```python
from build123d import *

# Parameters (mm, degrees)
SKETCH_1_W      = 26.2
SKETCH_1_H      = 15.4
SKETCH_1_R      = 1.5
SKETCH_1_W_2    = 25
SKETCH_1_H_2    = 2.55
EXTRUDE_1_DEPTH = 1.6
SKETCH_1_3_W    = 25
SKETCH_1_3_H    = 2.55
EXTRUDE_2_DEPTH = 2.65
SKETCH_2_W      = 0.628205128
SKETCH_2_H      = 3.5
EXTRUDE_3_DEPTH = 1.7


with BuildPart() as part:
    # Sketch 1 → Extrude 1 (new body)
    # profile 1 of 2: a face of its own
    with BuildSketch(Plane(origin=(0, 0, 0), x_dir=(1, 0, 0), z_dir=(0, 1, 0))):
        Rectangle(SKETCH_1_W, SKETCH_1_H)
        with Locations(Location((-10.15, -5.1, 0), (0, 0, 270))):
            Circle(SKETCH_1_R, mode=Mode.SUBTRACT)
        with Locations(Location((10.15, -5.1, 0), (0, 0, 270))):
            Circle(SKETCH_1_R, mode=Mode.SUBTRACT)
        with Locations((0, 6.025)):
            Rectangle(SKETCH_1_W_2, SKETCH_1_H_2, mode=Mode.SUBTRACT)
    # profile 2 of 2: a face of its own
    with BuildSketch(Plane(origin=(0, 0, 0), x_dir=(1, 0, 0), z_dir=(0, 1, 0))):
        with Locations((0, 6.025)):
            Rectangle(SKETCH_1_W_2, SKETCH_1_H_2)
    extrude(amount=EXTRUDE_1_DEPTH)

    # Sketch 1_3 → Extrude 2 (add)
    with BuildSketch(Plane(origin=(0, 0, 0), x_dir=(1, 0, 0), z_dir=(0, 1, 0))):
        with Locations((0, 6.025)):
            Rectangle(SKETCH_1_3_W, SKETCH_1_3_H)
    extrude(amount=-EXTRUDE_2_DEPTH)

    # Sketch 2 → Extrude 3 (add)
    with BuildSketch(Plane(origin=(0, 1.6, 0), x_dir=(1, 0, 0), z_dir=(0, 1, 0))):
        Polygon((0.5, -1.5), (-0.5, -1.5), (-0.5, -5.5), (-1.2, -5.5), (0, -6.930104311), (1.2, -5.5), (0.5, -5.5), align=None)
        Polygon((5.5, -1.2), (6.930104311, 0), (5.5, 1.2), (5.5, 0.5), (1.5, 0.5), (1.5, -0.5), (5.5, -0.5), align=None)
        with Locations((-3.28532471, 3.544331345)):
            Rectangle(SKETCH_2_W, SKETCH_2_H)
        Polygon((-1.886586729, 5.294331345), (-1.23454346, 5.294331345), (-0.435965736, 2.853025255), (0.368220963, 5.294331345), (1.013954136, 5.294331345), (1.605700931, 1.794331345), (0.969783463, 1.794331345), (0.596085547, 4.004968364), (-0.131678877, 1.794331345), (-0.744459325, 1.794331345), (-1.468017018, 4.004968364), (-1.841013812, 1.794331345), (-2.477632402, 1.794331345), align=None)
        with BuildLine():
            Line((2.189034264, 5.294331345), (2.817239393, 5.294331345))
            Line((2.817239393, 5.294331345), (2.817239393, 3.017087755))
            add(Edge.make_bspline(
                [(2.817239393, 3.017087755), (2.817273551, 2.993478281), (2.817339529, 2.947876826), (2.82064238, 2.882453669), (2.823664717, 2.822316089), (2.82911787, 2.767529925), (2.837174047, 2.71807174), (2.844975055, 2.673623833), (2.855532948, 2.634981994), (2.871399773, 2.590997464), (2.895845342, 2.541578443), (2.935788046, 2.490072805), (2.981878508, 2.443066435), (3.037120582, 2.403940113), (3.099207788, 2.372290446), (3.167798984, 2.348841544), (3.242797481, 2.335807069), (3.294654828, 2.333817117), (3.321345963, 2.332792883)],
                knots=[0, 0, 0, 0, 1.155499968, 2.231836252, 3.205919964, 4.102923608, 4.924856345, 5.658536265, 6.31071849, 6.882491295, 7.94666036, 8.992281882, 10.060072772, 11.158554251, 12.289267114, 13.461410017, 14.693379945, 16, 16, 16, 16], degree=3))
            add(Edge.make_bspline(
                [(3.321345963, 2.332792883), (3.349702001, 2.333620333), (3.404991473, 2.33523372), (3.484516578, 2.351070858), (3.558197038, 2.376289005), (3.624472787, 2.412281729), (3.68327787, 2.455425316), (3.733055141, 2.504622525), (3.772339181, 2.55997148), (3.797943056, 2.611035105), (3.812318371, 2.658034726), (3.823093386, 2.700027104), (3.830992664, 2.749573953), (3.838159148, 2.805901493), (3.842465653, 2.869593167), (3.847135356, 2.940136761), (3.848846846, 3.018014951), (3.849138556, 3.072242996), (3.849290675, 3.100521249)],
                knots=[0, 0, 0, 0, 1.261321664, 2.459363699, 3.594844139, 4.716940403, 5.803436589, 6.833651888, 7.818396249, 8.814403945, 9.360733334, 10.004355033, 10.743453831, 11.592799886, 12.532235708, 13.585170094, 14.740740724, 16, 16, 16, 16], degree=3))
            Line((3.849290675, 3.100521249), (3.849290675, 5.294331345))
            Line((3.849290675, 5.294331345), (4.477495803, 5.294331345))
            Line((4.477495803, 5.294331345), (4.477495803, 3.20639064))
            add(Edge.make_bspline(
                [(4.477495803, 3.20639064), (4.477408565, 3.164089061), (4.477240816, 3.08274725), (4.474664688, 2.965853344), (4.469180577, 2.859089511), (4.464574557, 2.762424556), (4.455660331, 2.675988702), (4.446373798, 2.599412843), (4.434537313, 2.532968347), (4.416925335, 2.457329363), (4.386532275, 2.370233842), (4.337534678, 2.269947127), (4.275335399, 2.171760357), (4.201818961, 2.076753656), (4.118812177, 1.988495493), (4.028155486, 1.91101625), (3.931289197, 1.845477164), (3.827201127, 1.793480747), (3.71597986, 1.752927462), (3.596524945, 1.725677696), (3.46891784, 1.707267413), (3.380777201, 1.705498879), (3.335368399, 1.704587755)],
                knots=[0, 0, 0, 0, 1.170808336, 2.251350247, 3.235597562, 4.129743112, 4.929140599, 5.639994148, 6.264258765, 6.79612947, 7.788252245, 8.809469599, 9.879094798, 10.999557536, 12.129761673, 13.226370002, 14.293821979, 15.358369427, 16.438775801, 17.562147481, 18.744053101, 20, 20, 20, 20], degree=3))
            add(Edge.make_bspline(
                [(3.335368399, 1.704587755), (3.305197888, 1.705095937), (3.245672088, 1.706098571), (3.158128956, 1.714939179), (3.073501323, 1.727966912), (2.991948202, 1.746973032), (2.913186538, 1.771525389), (2.837237257, 1.801747631), (2.764382604, 1.837471182), (2.695030264, 1.878367463), (2.62926558, 1.92258975), (2.569160054, 1.971612016), (2.512645313, 2.021808881), (2.461354044, 2.075292841), (2.414901005, 2.131502406), (2.373381866, 2.190564964), (2.33685831, 2.252475271), (2.304411607, 2.318349254), (2.276640395, 2.391535053), (2.253228221, 2.474635914), (2.232774795, 2.568954362), (2.217575015, 2.67470289), (2.203794806, 2.791532964), (2.195072693, 2.919748944), (2.190509763, 3.059354507), (2.189538525, 3.156140151), (2.189034264, 3.20639064)],
                knots=[0, 0, 0, 0, 1.001158378, 1.975264943, 2.917723546, 3.841610987, 4.75185031, 5.653588123, 6.552117133, 7.442167995, 8.324307438, 9.179605724, 10.014504199, 10.831958861, 11.636465792, 12.43274043, 13.225645099, 14.020104002, 14.867201867, 15.819789774, 16.883317127, 18.068162734, 19.364263498, 20.787406516, 22.332041935, 24, 24, 24, 24], degree=3))
            Line((2.189034264, 3.20639064), (2.189034264, 5.294331345))
        make_face()
        Polygon((1.779131112, -4.434974289), (2.226887522, -4.434974289), (2.66913178, -5.114665128), (3.112224061, -4.434974289), (3.560404483, -4.434974289), (2.893009985, -5.458538659), (3.604501705, -6.551640956), (3.156745295, -6.551640956), (2.66913178, -5.801988178), (2.18024623, -6.551640956), (1.732065808, -6.551640956), (2.445253575, -5.458114647), align=None)
        Polygon((6.501577719, -0.872404796), (6.924317436, -0.872404796), (7.302111907, -1.614849374), (7.679906378, -0.872404796), (8.102646095, -0.872404796), (7.492069172, -2.072358055), (7.492069172, -2.989071463), (7.112154642, -2.989071463), (7.112154642, -2.072358055), align=None)
    extrude(amount=EXTRUDE_3_DEPTH)


solid = part.part
```
Geometry check sheet. Reference: the model listing, model coordinates, mm. A direction names the side the tool comes from. Give positions to 0.01 mm unless a question says otherwise; leave off trailing zeros. Order: outer loops, then holes, each group sorted by start corner. A loop starts at its lowest first (then second) coordinate and runs counter-clockwise, first axis right, second up. Notation, with made-up numbers: (-26.5, 15) - (7.5, 15) arc R20 ccw to (7.5, 40) - close; hole circle Ø3 at (8, 60). An arc over 180 degrees is marked (long way). Answer in a Markdown table with one row per item. Add a question column.
Q1. Cross-section at C-C, the plane z = -0.75. Enter the section's corners in (x, y).
Q2. Material ranges on probe 1 along X at (y, z) = (1.25, 5.1); probe 2 along Y at (x, z) = (1, -2.5); probe 3 along Z at (x, y) = (11, -0.3), recorded low to high. Write a range as from..to.
Q3. Mould release check, pull along Z, two halves, no side actions. Record for faces 5 (the flat face through (7.3, 3.3, 1.9)), 6 (the flat face through (0.24, 2.44, -2.92)), 7 (the flat face through (-0.608, 2.438, 6.205)): pulls with the +Z half, pulls with the -Z half, needs draft (parallel to the pull), parting line crosses it, or undercut.
Q4. Tool access check on faces 1 (the flat face through (0, 2, 1.5)), 2 (the flat face through (7.112, 2.4, 2.5)), 3 (the flat face through (1.5, 2, 0)), 4 (the flat face through (-3.599, 2, -4)). Record the directions out of +Z, -Z, +X, -X, +Y, -Y that give a thin tool (end or side, any length) a straight path to the whole face; none if there is none.
Q5. Cross-section at B-B, the plane x = -8. Enter the section's corners in (y, z).
Q6. Gauge pin test, flat ends, axial feed: pin 1 (0.5 mm diameter, centred on x = 7, y = 2.5, fed in from -Z); pin 2 (2 mm diameter, centred on x = 5.5, z = 3, fed in from +Y); pin 3 (5 mm diameter, centred on x = 3.5, z = 1.5, fed in from -Y); pin 4 (2.5 mm diameter, centred on x = -10.15, z = 5.1, fed in from -Y). Record the tip position at first contact, or that the pin passes through.
Q7. Cross-section at D-D, the plane y = -1.95. Enter the section's corners in (x, z), then the cut area to 4 significant figures.
Q8. Cross-section at A-A, the plane x = 10.15. Enter the section's corners in (y, z), then the cut area to 3 significant figures.
Check values:
| question | item | result |
|---|---|---|
| 1 | outline | (-13.1, 0) - (13.1, 0) - (13.1, 1.6) - (6.04, 1.6) - (6.04, 3.3) - (5.5, 3.3) - (5.5, 1.6) - (-13.1, 1.6) - close |
| 2 | probe 1 | x = -13.1..-11.65, -8.65..8.65, 11.65..13.1 |
| 2 | probe 2 | y = 0..3.3 |
| 2 | probe 3 | z = -7.3..-4.75 |
| 3 | face 5 | needs draft |
| 3 | face 6 | undercut |
| 3 | face 7 | pulls with the +Z half |
| 4 | face 1 | -X, +Y |
| 4 | face 2 | +Z, +Y |
| 4 | face 3 | +Z, -X, +Y |
| 4 | face 4 | +Z, -Z, -X, +Y |
| 5 | outline | (-2.65, -7.3) - (0, -7.3) - (0, -7.7) - (1.6, -7.7) - (1.6, 7.7) - (0, 7.7) - (0, -4.75) - (-2.65, -4.75) - close |
| 6 | pin 1 | stops at z = -0.15 |
| 6 | pin 2 | stops at y = 1.6 |
| 6 | pin 3 | stops at y = 0 |
| 6 | pin 4 | passes through |
| 7 | outline | (-12.5, -7.3) - (12.5, -7.3) - (12.5, -4.75) - (-12.5, -4.75) - close |
| 7 | area | 63.75 mm^2 |
| 8 | outline | (-2.65, -7.3) - (0, -7.3) - (0, -7.7) - (1.6, -7.7) - (1.6, 3.6) - (0, 3.6) - (0, -4.75) - (-2.65, -4.75) - close; (0, 6.6) - (1.6, 6.6) - (1.6, 7.7) - (0, 7.7) - close |
| 8 | area | 26.6 mm^2 |
